CAD build for the part. Positions are in the model's coordinates, mm. Face numbers are marked on the shaded views. A direction names the side the tool comes from. Give positions to 0.01 mm unless a question says otherwise; leave off trailing zeros. Write each loop counter-clockwise with the first axis right and the second up, starting at its lowest first coordinate (ties: lowest second). Pieces come first, ordered by that corner, then holes. Notation, with made-up numbers: M 61,22 L 75,22 A11 cw 75,37 Z; hole C 14.5,18 d10. An arc over 180 degrees is marked long. One line per question, with ' | ' between items. Start each with the question number.
1. Pull direction X, two halves, no side cores. Call the marked faces 1, 2 and 3: released by +X, released by -X, zero draft, split by the parting line, or undercut.
2. Cut at A-A, the plane x = 0. Write the cut outline in (y, z).
3. Cut at D-D, the plane z = 4. Write the cut outline in (x, y).
4. Which spindle directions (+Z, -Z, +X, -X, +Y, -Y) get a long thin tool onto all of the face, cutting with end or side? Do the marked faces 4, 5 and 6. Say none if no direction does.
5. Wall check: L1, parallel to Y at x = 0, z = 3.5; L2, parallel to Y at x = 5, z = 3.65; L3, parallel to X at y = -0.5, z = 0.65. Give the ranges that are in metal, low to high.
6. Cut at C-C, the plane x = -6. Write the cut outline in (y, z), then the cut area to 3 significant figures.
7. Cut at B-B, the plane y = -6.5. Write the cut outline in (x, z), then the cut area to 3 significant figures.
8. Flat gauge pins, fed straight in: pin 1 (1.5 mm diameter, centred on y = 0, z = 2.5, fed in from -X); pin 2 (3 mm diameter, centred on x = -3.5, z = 2, fed in from +Y); pin 3 (2.5 mm diameter, centred on x = 0, y = 6.5, fed in from -Z). Where does each tip first touch, or does it go through?
```python
from build123d import *

# Parameters (mm, degrees)
SKETCH_1_R          = 8.5
EXTRUDE_1_DEPTH     = 5
SKETCH_2_R          = 1.5
CUT_EXTRUDE_1_DEPTH = 5
CUT_EXTRUDE_2_DEPTH = 6
EXTRUDE_2_DEPTH     = 5
FILLET_2_R          = 0.5
CUT_EXTRUDE_3_DEPTH = 10
FILLET_3_R          = 0.5


with BuildPart() as part:
    # 草图1 → 凸台-拉伸1 (new body)
    with BuildSketch(Plane.XY):
        Circle(SKETCH_1_R)
    extrude(amount=EXTRUDE_1_DEPTH)

    # 草图2 → 切除-拉伸1 (cut)
    with BuildSketch(Plane.XY.offset(5)):
        with Locations((0, 6.5)):
            Circle(SKETCH_2_R)
        with Locations((0, -6.5)):
            Circle(SKETCH_2_R)
    extrude(amount=-CUT_EXTRUDE_1_DEPTH, mode=Mode.SUBTRACT)

    # 草图3 → 切除-拉伸2 (cut, through all)
    with BuildSketch(Plane(origin=(0, 0, 0), x_dir=(-1, 0, 0), z_dir=(0, 0, -1))):
        with BuildLine():
            Line((6.962792376, 4.875399709), (3.89097221, 2.724488073))
            ThreePointArc((3.89097221, 2.724488073), (4.530155516, 1.428352548), (4.75, 0))
            ThreePointArc((4.75, 0), (4.530155516, -1.428352548), (3.89097221, -2.724488073))
            Line((3.89097221, -2.724488073), (6.962792376, -4.875399709))
            ThreePointArc((6.962792376, -4.875399709), (8.106594081, -2.555999296), (8.5, 0))
            ThreePointArc((8.5, 0), (8.106594081, 2.555999296), (6.962792376, 4.875399709))
        make_face()
    cut_extrude_2 = extrude(amount=-CUT_EXTRUDE_2_DEPTH, mode=Mode.SUBTRACT)

    # 镜向1: 切除-拉伸2 across plane
    add(cut_extrude_2.mirror(Plane(origin=(0, 0, 0), x_dir=(0, 0, 1), z_dir=(1, 0, 0))), mode=Mode.SUBTRACT)


with BuildPart() as body_2:
    # 草图4 → 凸台-拉伸2 (new body)
    with BuildSketch(Plane(origin=(0, 0, 0), x_dir=(-1, 0, 0), z_dir=(0, 0, -1))):
        with BuildLine():
            ThreePointArc((6.962792376, -4.875399709), (0, -8.5), (-6.962792376, -4.875399709))
            Line((-6.962792376, -4.875399709), (-6.962792376, -20))
            Line((-6.962792376, -20), (6.962792376, -20))
            Line((6.962792376, -20), (6.962792376, -4.875399709))
        make_face()
    extrude(amount=-EXTRUDE_2_DEPTH)


with BuildPart() as part_1:
    add(part.part)

    # Combine 1: union body 2
    add(body_2.part)

    # 圆角2
    fillet_2_edges = [part_1.edges().sort_by_distance(p)[0] for p in [
        (-6.962792376, -20, 2.5),
        (6.962792376, -20, 2.5),
    ]]
    fillet(fillet_2_edges, radius=FILLET_2_R)

    # 草图6 → 切除-拉伸3 (cut)
    with BuildSketch(Plane(origin=(0, 0, 0), x_dir=(-1, 0, 0), z_dir=(0, 0, -1))):
        with BuildLine():
            Line((3.89097221, 2.724488073), (3.89097221, -2.724488073))
            ThreePointArc((3.89097221, -2.724488073), (4.75, 0), (3.89097221, 2.724488073))
        make_face()
        with BuildLine():
            Line((-3.89097221, 2.724488073), (-3.89097221, -2.724488073))
            ThreePointArc((-3.89097221, -2.724488073), (-4.75, 0), (-3.89097221, 2.724488073))
        make_face()
    extrude(amount=-CUT_EXTRUDE_3_DEPTH, mode=Mode.SUBTRACT)

    # 圆角3
    fillet_3_edges = [part_1.edges().sort_by_distance(p)[0] for p in [
        (-3.89097221, -2.724488073, 2.5),
        (-3.89097221, 2.724488073, 2.5),
        (3.89097221, 2.724488073, 2.5),
        (3.89097221, -2.724488073, 2.5),
    ]]
    fillet(fillet_3_edges, radius=FILLET_3_R)


solid = part_1.part
```
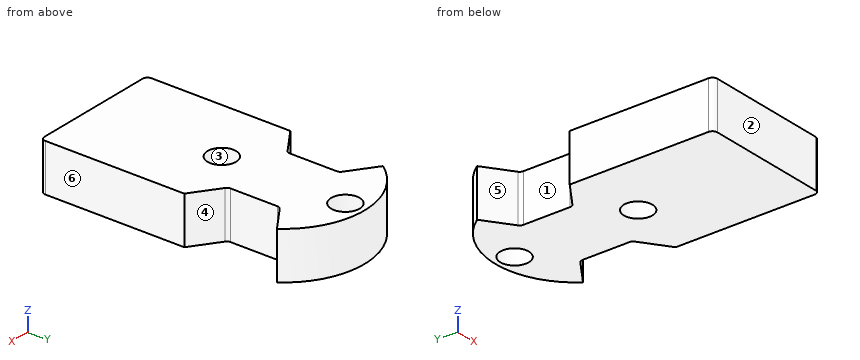
Here are the results:
1) face 1: released by -X | face 2: zero draft | face 3: undercut
2) outline: M -20,0 L -8,0 L -8,5 L -20,5 Z; M -5,0 L 5,0 L 5,5 L -5,5 Z; M 8,0 L 8.5,0 L 8.5,5 L 8,5 Z
3) outline: M -6.96,-19.5 A0.5 ccw -6.46,-20 L 6.46,-20 A0.5 ccw 6.96,-19.5 L 6.96,-4.88 L 4.1,-2.87 A0.5 cw 3.89,-2.46 L 3.89,2.46 A0.5 cw 4.1,2.87 L 6.96,4.88 A8.5 ccw -6.96,4.88 L -4.1,2.87 A0.5 cw -3.89,2.46 L -3.89,-2.46 A0.5 cw -4.1,-2.87 L -6.96,-4.88 Z; hole C 0,-6.5 d3; hole C 0,6.5 d3
4) face 4: +Z, -Z, +X | face 5: +Z, -Z, -X | face 6: +Z, -Z, +X, +Y, -Y
5) L1: -20 to -8, -5 to 5, 8 to 8.5 | L2: -20 to -3.5, 3.5 to 6.87 | L3: -3.89 to 3.89
6) outline: M -20,0 L -4.2,0 L -4.2,5 L -20,5 Z; M 4.2,0 L 6.02,0 L 6.02,5 L 4.2,5 Z | area: 88.1 mm^2
7) outline: M -6.96,0 L -1.5,0 L -1.5,5 L -6.96,5 Z; M 1.5,0 L 6.96,0 L 6.96,5 L 1.5,5 Z | area: 54.6 mm^2
8) pin 1: x = -3.89 | pin 2: y = 8.26 | pin 3: through
